Read the model definition and answer for the solid it produces. Units are mm, in the model's axes. Face numbers are marked on the shaded views. A direction names the side the tool comes from. Give positions to 0.01 mm unless a question says otherwise; leave off trailing zeros. Loops run counter-clockwise (first coordinate to the right, second up) from the corner with the lowest first, then second, coordinate; pieces in that order, holes last. Notation, with made-up numbers: (21.5, -18.5) -> (29.5, -18.5) arc R15 ccw to (29.5, -1.5) -> close; hole circle Ø6 at (35.25, 8.25). An arc over 180 degrees is marked (long way). Write each question's results on one line, items separated by ' | '. Start each with the question number.
Item 1: Section C-C on z = 7.5 is taken. State how many separate pieces and enclosed holes the cut face has, and give its area (3 significant figures).
Item 2: Each of these flat-tipped pins is pushed along its axis until it touches: P1, Ø3.5, axis at x = 0, y = 69, coming from the -Z side; P2, Ø3, axis at x = -25.5, z = 4, coming from the +Y side; P3, Ø6, axis at y = -25.5, z = 14, coming from the +X side; P4, Ø12, axis at x = 34, z = 2, coming from the +Y side. Where does it stop, or does it pass through?
Item 3: Section D-D on y = 69 is taken. Write down the section's boundary in (x, z).
Item 4: Section B-B on x = 23 is taken. Write down the section's boundary in (y, z).
Item 5: Section A-A on y = 0 is taken. Write down the section's boundary in (x, z), and give its area (3 significant figures).
Item 6: Find the intervals of material crossed by line 1 (Y direction, x = 0, z = 17.95); line 2 (Y direction, x = 0, z = 11.5); line 3 (Y direction, x = 1, z = 13.5), in increasing order.
Item 7: Which of the six approach directions +Z, -Z, +X, -X, +Y, -Y give full straight-line access (tool end or side, diameter ignored) to the marked faces 1 and 2?
Item 8: Determine the mould class of the marked faces 3, 4 and 5 for opening direction X: +X half, -X half, draft (parallel to the pull), parting line (faces both ways), or undercut.
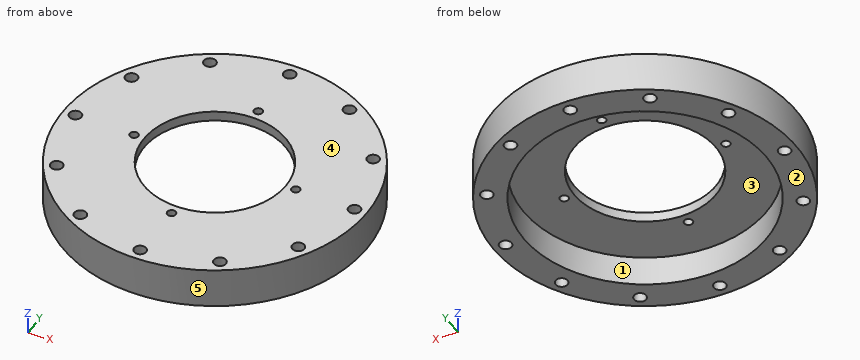
```python
from build123d import *

# Parameters (mm, degrees)
SKETCH_1_R          = 75
SKETCH_1_R_2        = 35
SKETCH_1_R_3        = 3
EXTRUDE_1_DEPTH     = 20
SKETCH_2_R          = 60
CUT_EXTRUDE_1_DEPTH = 15
HOLE_WIZARD_M5_2_D  = 4.2


with BuildPart() as part:
    # 草图1 → 凸台-拉伸1 (new body)
    with BuildSketch(Plane.XY):
        Circle(SKETCH_1_R)
        Circle(SKETCH_1_R_2, mode=Mode.SUBTRACT)
        with Locations((-69, 0)):
            Circle(SKETCH_1_R_3, mode=Mode.SUBTRACT)
        with Locations((-59.755752861, 34.5)):
            Circle(SKETCH_1_R_3, mode=Mode.SUBTRACT)
        with Locations((-34.5, 59.755752861)):
            Circle(SKETCH_1_R_3, mode=Mode.SUBTRACT)
        with Locations((0, 69)):
            Circle(SKETCH_1_R_3, mode=Mode.SUBTRACT)
        with Locations((34.5, 59.755752861)):
            Circle(SKETCH_1_R_3, mode=Mode.SUBTRACT)
        with Locations((59.755752861, 34.5)):
            Circle(SKETCH_1_R_3, mode=Mode.SUBTRACT)
        with Locations((69, 0)):
            Circle(SKETCH_1_R_3, mode=Mode.SUBTRACT)
        with Locations((59.755752861, -34.5)):
            Circle(SKETCH_1_R_3, mode=Mode.SUBTRACT)
        with Locations((34.5, -59.755752861)):
            Circle(SKETCH_1_R_3, mode=Mode.SUBTRACT)
        with Locations((0, -69)):
            Circle(SKETCH_1_R_3, mode=Mode.SUBTRACT)
        with Locations((-34.5, -59.755752861)):
            Circle(SKETCH_1_R_3, mode=Mode.SUBTRACT)
        with Locations((-59.755752861, -34.5)):
            Circle(SKETCH_1_R_3, mode=Mode.SUBTRACT)
    extrude(amount=EXTRUDE_1_DEPTH)

    # 草图2 → 切除-拉伸1 (cut)
    with BuildSketch(Plane.XY):
        Circle(SKETCH_2_R)
    extrude(amount=CUT_EXTRUDE_1_DEPTH, mode=Mode.SUBTRACT)

    # M5 螺纹孔的螺纹孔钻头2 (through all)
    with Locations(Plane.XY.offset(20)):
        with Locations((0, 40), (40, 0), (0, -40), (-40, 0)):
            Hole(HOLE_WIZARD_M5_2_D / 2)


solid = part.part
```
Findings:
1) separate pieces: 1 | enclosed holes: 13 | area: 6,020 mm2
2) P1: through | P2: y = 71.06 | P3: x = 71.55 | P4: y = 69.58
3) outline: (-29.39, 0) -> (-3, 0) -> (-3, 20) -> (-29.39, 20) -> close; (3, 0) -> (29.39, 0) -> (29.39, 20) -> (3, 20) -> close
4) outline: (-71.39, 0) -> (-55.42, 0) -> (-55.42, 15) -> (-26.38, 15) -> (-26.38, 20) -> (-71.39, 20) -> close; (26.38, 15) -> (55.42, 15) -> (55.42, 0) -> (71.39, 0) -> (71.39, 20) -> (26.38, 20) -> close
5) outline: (-75, 0) -> (-72, 0) -> (-72, 20) -> (-75, 20) -> close; (-66, 0) -> (-60, 0) -> (-60, 15) -> (-42.1, 15) -> (-42.1, 20) -> (-66, 20) -> close; (-37.9, 15) -> (-35, 15) -> (-35, 20) -> (-37.9, 20) -> close; (35, 15) -> (37.9, 15) -> (37.9, 20) -> (35, 20) -> close; (42.1, 15) -> (60, 15) -> (60, 0) -> (66, 0) -> (66, 20) -> (42.1, 20) -> close; (72, 0) -> (75, 0) -> (75, 20) -> (72, 20) -> close | area: 568 mm2
6) line 1: -75 to -72, -66 to -42.1, -37.9 to -35, 35 to 37.9, 42.1 to 66, 72 to 75 | line 2: -75 to -72, -66 to -60, 60 to 66, 72 to 75 | line 3: -74.99 to -71.83, -66.17 to -59.99, 59.99 to 66.17, 71.83 to 74.99
7) face 1: -Z | face 2: -Z, +X, -X, +Y, -Y
8) face 3: undercut | face 4: draft | face 5: parting line
